Autodesk Fusion 360 part; units mm, degrees
sketch "Sketch1" plane through (0, 0, 0) normal (0, 0, 1) x (1, 0, 0)
  line L0 (0, 0) -> (-42, 0)
  line L1 (-42, 0) -> (-42, 10)
  line L2 (-42, 10) -> (0, 10)
  line L3 (0, 10) -> (0, 0)
  line L4 (3.6, -3.6) -> (-45.6, -3.6)
  line L5 (-45.6, -3.6) -> (-45.6, 13.6)
  line L6 (-45.6, 13.6) -> (3.6, 13.6)
  line L7 (3.6, 13.6) -> (3.6, -3.6)
  dimension "d1" = 42
  dimension "d2" = 10
  dimension "d3" = -3.6
extrude "Extrude1" add sketch "Sketch1" along normal blind 65
extrude "Extrude2" add sketch "Sketch1" against normal blind 5 contours L0 L1 L2 L3 | L4 L5 L6 L7
sketch "Sketch2" plane through (0, -3.6, 0) normal (0, -1, 0) x (1, 0, 0)
  line L0 (3.6, -5) -> (3.6, 65)
  line L1 (3.6, 65) -> (-45.6, 65)
  line L2 (-45.6, 65) -> (-45.6, -5)
  line L3 (-45.6, -5) -> (3.6, -5)
  curve L4
  curve L5
  line L6 (-21, 65) -> (-21, -5)
  spline S0 degree 2 poles (-42, 65) (-21, 34) (0, 65) knots 0 0 0 5.982089 5.982089 5.982089 weights 1 2.19545 1
  point P0 (0, 65)
  point P1 (-42, 65)
extrude "Extrude3" cut sketch "Sketch2" against normal blind 13.6 contours L1 L6 S0 | L1 L6 S0
fillet "Fillet1" radius 4.5 3 edges at (-45.6, -3.6, 30) (-21, -3.6, -5) (3.6, -3.6, 30)
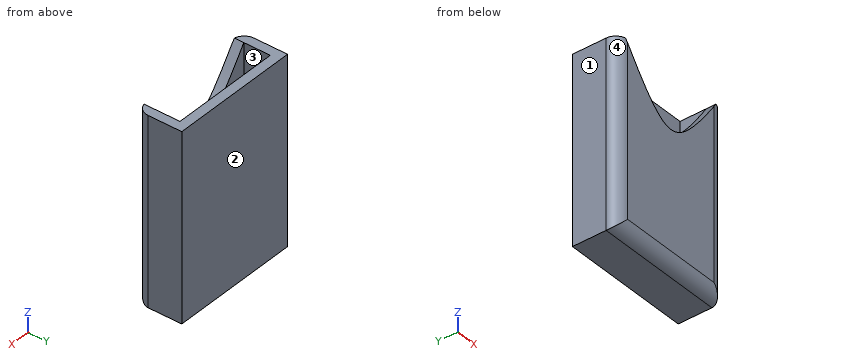
Work out the finished part from the listing and answer in its coordinate system (mm). Face numbers are marked on the shaded views. Give positions to 0.01 mm unless a question says otherwise; leave off trailing zeros. Write each loop counter-clockwise with the first axis right and the second up, starting at its lowest first coordinate (ties: lowest second). Pieces come first, ordered by that corner, then holes.
Q1. The part is cut by section B-B on y = 3. Give the vertices of the cut face in (x, z).
Answer:
outline: (-45.6, -5) - (3.6, -5) - (3.6, 65) - (0, 65) - (0, 0) - (-42, 0) - (-42, 65) - (-45.6, 65) - close
Q2. Straight lines are drawn through the part: L1, parallel to Y at x = -0.5, z = 32; L2, parallel to X at y = 4.5, z = 9.5; L3, parallel to Z at x = -33.5, y = 9.25. For each, find the intervals that lie inside material, in ascending order.
Answer:
L1: y = -3.58 to 0, 10 to 13.6
L2: x = -45.6 to -42, 0 to 3.6
L3: z = -5 to 0
Q3. For a pull along Y with two mould halves and no side action, classify the marked faces 1, 2, 3 and 4 as released by +Y, released by -Y, zero draft, split by the parting line, or undercut.
Answer:
face 1: zero draft
face 2: released by +Y
face 3: undercut
face 4: released by -Y
Q4. Given pin 1 (1 mm diameter, centred on y = -1, z = 47.5, fed in from +X); pin 2 (3 mm diameter, centred on x = -34.5, y = 0, fed in from -Z), each flat-ended and moving along its own axis, determine where each tip first touches the part or whether it passes through.
Answer:
pin 1: stops at x = 3.38
pin 2: stops at z = -5
Q5. The part is cut by section A-A on z = 41. Give the vertices of the cut face in (x, y).
Answer:
outline: (-45.6, 0.9) arc R4.5 ccw to (-41.1, -3.6) - (-0.9, -3.6) arc R4.5 ccw to (3.6, 0.9) - (3.6, 13.6) - (-45.6, 13.6) - close; hole (-42, 0) - (0, 0) - (0, 10) - (-42, 10) - close
